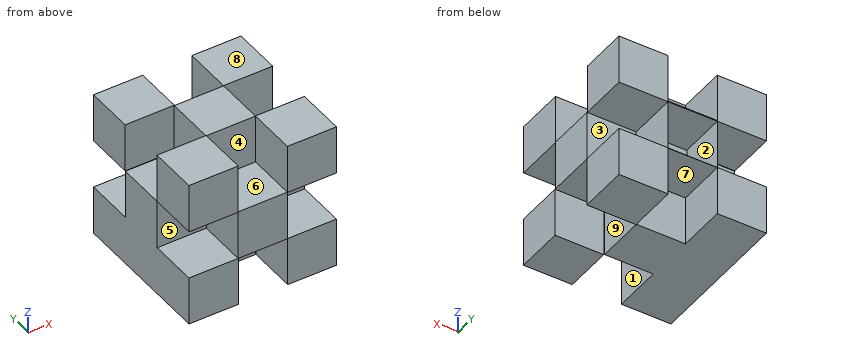
```python
from build123d import *

# Parameters (mm, degrees)
F0_W      = 76.2
F0_H      = 76.2
F1_DEPTH  = 76.2
F3_W      = 25.4
F3_H      = 25.4
F4_W      = 25.4
F4_H      = 25.4
F5_W      = 25.4
F5_H      = 25.4
F6_W      = 25.4
F6_H      = 25.4
F7_DEPTH  = 25.4
F14_W     = 25.4
F14_H     = 25.4
F13_W     = 25.4
F13_H     = 25.4
F12_W     = 25.4
F12_H     = 25.4
F11_W     = 25.4
F11_H     = 25.4
F15_DEPTH = 25.4
F16_W     = 25.4
F16_H     = 25.4
F17_W     = 25.4
F17_H     = 25.4
F18_DEPTH = 25.4
F20_W     = 25.4
F20_H     = 25.4
F21_DEPTH = 25.4
F2_W      = 25.4
F2_H      = 25.4
F22_DEPTH = 24.384


with BuildPart() as f1:
    # F0 (on Front) → F1 (new body)
    with BuildSketch(Plane.XZ):
        Rectangle(F0_W, F0_H)
    extrude(amount=F1_DEPTH)

    # F3 (on Front) + F4 (on Front) + F5 (on Front) + F6 (on Front) → F7 (cut)
    with BuildSketch(Plane.XZ):
        with Locations((-25.449485, 0.03107)):
            Rectangle(F3_W, F3_H)
    with BuildSketch(Plane.XZ):
        with Locations((0.029016, 25.827004)):
            Rectangle(F4_W, F4_H)
    with BuildSketch(Plane.XZ):
        with Locations((25.474846, -0.000868)):
            Rectangle(F5_W, F5_H)
    with BuildSketch(Plane.XZ):
        with Locations((0.018974, -25.553884)):
            Rectangle(F6_W, F6_H)
    extrude(amount=F7_DEPTH, mode=Mode.SUBTRACT)

    # F14 (on offset) + F13 (on offset) + F12 (on offset) + F11 (on offset) → F15 (cut)
    with BuildSketch(Plane.XZ.offset(76.2)):
        with Locations((-25.426297, -0.069618)):
            Rectangle(F14_W, F14_H)
    with BuildSketch(Plane.XZ.offset(76.2)):
        with Locations((0.216928, -25.486759)):
            Rectangle(F13_W, F13_H)
    with BuildSketch(Plane.XZ.offset(76.2)):
        with Locations((25.516777, -0.001813)):
            Rectangle(F12_W, F12_H)
    with BuildSketch(Plane.XZ.offset(76.2)):
        with Locations((0.029588, 25.589703)):
            Rectangle(F11_W, F11_H)
    extrude(amount=-F15_DEPTH, mode=Mode.SUBTRACT)

    # F16 (on offset) + F17 (on offset) → F18 (cut)
    with BuildSketch(Plane.YZ.offset(38.1)):
        with Locations((-37.974666, 25.560617)):
            Rectangle(F16_W, F16_H)
    with BuildSketch(Plane.YZ.offset(38.1)):
        with Locations((-38.356981, -25.470397)):
            Rectangle(F17_W, F17_H)
    extrude(amount=-F18_DEPTH, mode=Mode.SUBTRACT)

    # F20 (on offset) → F21 (cut)
    with BuildSketch(Plane.XY.offset(38.1)):
        with Locations((-25.548159, -37.909492)):
            Rectangle(F20_W, F20_H)
    extrude(amount=-F21_DEPTH, mode=Mode.SUBTRACT)

    # F2 (on Front) → F22 (cut)
    with BuildSketch(Plane.XZ):
        Rectangle(F2_W, F2_H)
    extrude(amount=F22_DEPTH, mode=Mode.SUBTRACT)


solid = f1.part
```
Verification items for the finished model (mm, model axes). Face numbers are marked on the shaded views. A direction names the side the tool comes from. Give positions to 0.01 mm unless a question says otherwise; leave off trailing zeros. Order: outer loops, then holes, each group sorted by start corner. A loop starts at its lowest first (then second) coordinate and runs counter-clockwise, first axis right, second up. Notation, with made-up numbers: M 35,-17.5 L 45,-17.5 A31 cw 45,8.5 Z; hole C 6.25,82.25 d10. An arc over 180 degrees is marked long. Return JSON: item names as keys, results as strings. Group by question number.
1) Section check B-B on z = 26. Record the cut outline in (x, y), and give its area (3 significant figures).
2) Access from +Z, -Z, +X, -X, +Y, -Y to the whole of each face (thin tool, end or side, straight path). Record for the marked faces 1, 2, 3, 4 and 5.
3) Go/stop test with flat-tipped pins: pin 1 Ø12.5 at (y, z) = (-41, -28.5) entering from +X; pin 2 Ø12.5 at (x, z) = (0, -27.5) entering from +Y; pin 3 Ø12.5 at (y, z) = (-67.5, 1) entering from -X. Record where each tip stops, or that it passes through.
4) Section check A-A on x = -17.5. Record the cut outline in (y, z), and give its area (3 significant figures).
5) Section check C-C on y = -16. Record the cut outline in (x, z), and give its area (3 significant figures).
6) Section check D-D on y = -48. Record the cut outline in (x, z), and give its area (3 significant figures).
7) Scan lines: line 1 (Y direction, x = 24, z = 19.5); line 2 (Y direction, x = -15, z = 30.5); line 3 (X direction, y = -8.5, z = -22). Record each from-to range of solid material in increasing order.
8) Mould release check, pull along X, two halves, no side actions. Record for the marked faces 6, 7, 8 and 9: pulls with the +X half, pulls with the -X half, needs draft (parallel to the pull), parting line crosses it, or undercut.
Answer block:
{
 "1": {"outline": "M -38.1,-76.2 L -12.67,-76.2 L -12.67,-50.8 L 12.73,-50.8 L 12.73,-76.2 L 38.1,-76.2 L 38.1,-50.67 L 12.7,-50.67 L 12.7,-25.4 L -12.67,-25.4 L -12.67,0 L -38.1,0 L -38.1,-25.21 L -12.85,-25.21 L -12.85,-50.61 L -38.1,-50.61 Z; M 12.73,-25.27 L 38.1,-25.27 L 38.1,0 L 12.73,0 Z", "area": "3,230 mm^2"},
 "2": {"face 1": "-Z, -Y", "face 2": "+Y", "face 3": "+X, +Y", "face 4": "+Z, -Y", "face 5": "-X, -Y"},
 "3": {"pin 1": "stops at x = 12.7", "pin 2": "stops at y = -25.4", "pin 3": "stops at x = -12.73"},
 "4": {"outline": "M -76.2,-38.1 L 0,-38.1 L 0,-12.67 L -25.4,-12.67 L -25.4,12.7 L -50.61,12.7 L -50.61,38.1 L -76.2,38.1 L -76.2,12.63 L -50.8,12.63 L -50.8,-12.77 L -76.2,-12.77 Z; M -25.21,12.73 L 0,12.73 L 0,38.1 L -25.21,38.1 Z", "area": "3,870 mm^2"},
 "5": {"outline": "M -38.1,-38.1 L -12.68,-38.1 L -12.68,-12.85 L 12.72,-12.85 L 12.72,-38.1 L 38.1,-38.1 L 38.1,-12.7 L 12.77,-12.7 L 12.77,12.7 L 38.1,12.7 L 38.1,38.1 L 12.73,38.1 L 12.73,13.13 L -12.67,13.13 L -12.67,38.1 L -38.1,38.1 L -38.1,12.73 L -12.75,12.73 L -12.75,-12.67 L -38.1,-12.67 Z; hole M -12.7,-12.7 L 12.7,-12.7 L 12.7,12.7 L -12.7,12.7 Z", "area": "2,600 mm^2"},
 "6": {"outline": "M -38.1,-38.1 L 12.7,-38.1 L 12.7,-12.77 L 38.1,-12.77 L 38.1,12.86 L 12.7,12.86 L 12.7,38.1 L -12.85,38.1 L -12.85,12.7 L -38.1,12.7 Z", "area": "3,880 mm^2"},
 "7": {"line 1": "y = -76.2 to -50.67, -25.27 to 0", "line 2": "y = -76.2 to -50.61, -25.21 to 0", "line 3": "x = -38.1 to -12.68, 12.72 to 38.1"},
 "8": {"face 6": "undercut", "face 7": "undercut", "face 8": "needs draft", "face 9": "pulls with the +X half"}
}
